Autodesk Inventor part; units mm, degrees
ref_plane "YZ Plane" through (0, 0, 0) normal (1, 0, 0) x (0, 1, 0)
ref_plane "XZ Plane" through (0, 0, 0) normal (0, 1, 0) x (-1, 0, 0)
ref_plane "XY Plane" through (0, 0, 0) normal (0, 0, 1) x (1, 0, 0)
sketch "Esquisse1" plane through (0, 0, 0) normal (0, 1, 0) x (-1, 0, 0)
  line L0 (21, 10.5) -> (-21, 10.5)
  line L1 (-21, 10.5) -> (-21, -10.5)
  line L2 (-21, -10.5) -> (21, -10.5)
  line L3 (21, -10.5) -> (21, 10.5)
  line L4 (29, 12.5) -> (-29, 12.5)
  line L5 (-29, 12.5) -> (-29, -12.5)
  line L6 (-29, -12.5) -> (29, -12.5)
  line L7 (29, -12.5) -> (29, 12.5)
  point P0 (0, 0)
  dimension "d0" = 21
  dimension "d1" = 10.5
  dimension "d2" = 42
  dimension "d3" = 21
  dimension "d4" = 2
  dimension "d5" = 2
  dimension "d6" = 8
  dimension "d7" = 8
extrude "Extrusion1" add sketch "Esquisse1" along normal blind 28
sketch "Esquisse2" plane through (0, 28, 0) normal (0, 1, 0) x (1, 0, 0)
  line L0 (-29, -12.5) -> (29, -12.5)
  line L1 (29, -12.5) -> (29, 12.5)
  line L2 (29, 12.5) -> (-29, 12.5)
  line L3 (-29, 12.5) -> (-29, -12.5)
  point P0 (0, 0)
extrude "Extrusion2" add sketch "Esquisse2" along normal blind 5
sketch "Esquisse3" plane through (0, 0, 0) normal (0, -1, 0) x (1, 0, 0)
  line L0 (-28, 10.5) -> (-21, 0) construction
  line L1 (-21, 0) -> (-28, -10.5) construction
  line L2 (-21, -10.5) -> (-28, 0) construction
  line L3 (-28, 0) -> (-21, 10.5) construction
  line L4 (21, 10.5) -> (28, 0) construction
  line L5 (21, -10.5) -> (28, 0) construction
  line L6 (28, -10.5) -> (21, 0) construction
  line L7 (21, 0) -> (28, 10.5) construction
  circle A0 centre (24.5, 5.25) radius 2
  circle A1 centre (24.5, -5.25) radius 2
  circle A2 centre (-24.5, 5.25) radius 2
  circle A3 centre (-24.5, -5.25) radius 2
  line L8 (-21, 10.5) -> (-28, 10.5)
  line L9 (-28, 10.5) -> (-28, -10.5)
  line L10 (-28, -10.5) -> (-21, -10.5)
  line L11 (-21, -10.5) -> (-21, 10.5)
  line L12 (28, 10.5) -> (21, 10.5)
  line L13 (21, 10.5) -> (21, -10.5)
  line L14 (21, -10.5) -> (28, -10.5)
  line L15 (28, -10.5) -> (28, 10.5)
  line L16 (21, 10.5) -> (21, -10.5)
  line L17 (21, -10.5) -> (-21, -10.5)
  line L18 (-21, 10.5) -> (21, 10.5)
  line L19 (-21, -10.5) -> (-21, 10.5)
  point P0 (0, 0)
  dimension "d12" = 4
  dimension "d13" = 4
  dimension "d14" = 4
  dimension "d15" = 4
  dimension "d25" = 7
  dimension "d26" = 7
extrude "Extrusion3" cut sketch "Esquisse3" against normal through all contours A0 | A1 | A2 | A3
sketch "Esquisse4" plane through (0, 28, 0) normal (0, -1, 0) x (1, 0, 0)
  line L0 (-21, 10.5) -> (10, 10.5)
  line L1 (10, 10.5) -> (10, -10.5)
  line L2 (10, -10.5) -> (-21, -10.5)
  line L3 (-21, -10.5) -> (-21, 10.5)
  line L4 (21, -10.5) -> (-21, -10.5)
  circle A0 centre (10, 0) radius 3.5
  line L5 (21, 10.5) -> (21, -10.5)
  point P0 (0, 0)
  dimension "d19" = 7
  dimension "d50" = 11
extrude "Extrusion4" cut sketch "Esquisse4" against normal through all contours A0 L1 | L1 A0
chamfer "Chanfrein1" distance 3 angle 45 1 edges at (6.5, 28, 0)
sketch "Esquisse5" plane through (-29, 0, 12.5) normal (0, 0, 1) x (1, 0, 0)
  line L0 (0, 0) -> (25, 0)
  line L1 (25, 0) -> (25, 19)
  line L2 (25, 19) -> (0, 19)
  line L3 (0, 19) -> (0, 0)
  line L4 (25, 0) -> (58, 0)
  line L5 (58, 0) -> (58, 6)
  line L6 (58, 6) -> (25, 6)
  line L7 (25, 6) -> (25, 0)
  line L8 (25, 19) -> (38, 6)
  point P0 (29, 0)
  dimension "d27" = 19
  dimension "d29" = 6
  dimension "d30" = 45
  dimension "d33" = 20
extrude "Extrusion5" cut sketch "Esquisse5" against normal through all
sketch "Esquisse6" plane through (0, 33, 0) normal (0, 1, 0) x (1, 0, 0)
  circle A0 centre (-24.5, -5.25) radius 4
  circle A1 centre (-24.5, 5.25) radius 4
  circle A2 centre (24.5, -5.25) radius 4
  circle A3 centre (24.5, 5.25) radius 4
  circle A4 centre (24.5, 5.25) radius 2
  circle A5 centre (24.5, -5.25) radius 2
  circle A6 centre (-24.5, -5.25) radius 2
  circle A7 centre (-24.5, 5.25) radius 2
  point P0 (0, 0)
  dimension "d34" = 8
  dimension "d35" = 8
  dimension "d36" = 8
  dimension "d37" = 8
extrude "Extrusion6" cut sketch "Esquisse6" against normal blind 13
sketch "Esquisse7" plane through (29, 33, 12.5) normal (1, 0, 0) x (0, 0, -1)
  line L0 (7.5, -27) -> (17.5, -27)
  line L1 (17.5, -27) -> (17.5, -5)
  line L2 (17.5, -5) -> (7.5, -5)
  line L3 (7.5, -5) -> (7.5, -27)
  line L4 (0, -27) -> (25, -27)
  line L5 (15.8135, -5) -> (9.1865, -5)
  line L6 (17.5, -27) -> (15.5, -27)
  line L7 (15.5, -27) -> (15.5, -17)
  line L8 (15.5, -17) -> (17.5, -17)
  line L9 (17.5, -17) -> (17.5, -27)
  line L10 (7.5, -27) -> (9.5, -27)
  line L11 (9.5, -27) -> (9.5, -17)
  line L12 (9.5, -17) -> (7.5, -17)
  line L13 (7.5, -17) -> (7.5, -27)
  point P0 (12.5, -33)
  dimension "d40" = 10
  dimension "d41" = 5
  dimension "d44" = 6
  dimension "d45" = 3
  dimension "d46" = 10
extrude "Extrusion7" cut sketch "Esquisse7" against normal up to next contours L11 L12 L3 L2 L1 L8 L7 L0
chamfer "Chanfrein2" distance 2 angle 45 2 edges at (25, 16, 3) (25, 16, -3)
sketch "Esquisse8" plane through (0, 28, 0) normal (0, -1, 0) x (1, 0, 0)
  line L0 (-16, -5.5) -> (-1.5, -5.5)
  line L1 (-1.5, -5.5) -> (-1.5, 5.5)
  line L2 (-1.5, 5.5) -> (-16, 5.5)
  line L3 (-16, 5.5) -> (-16, -5.5)
  line L4 (-21, 3.3135) -> (-21, -3.3135)
  line L5 (-4, 10.5) -> (-21, 10.5)
  line L6 (-21, -10.5) -> (-4, -10.5)
  circle A0 centre (10, 0) radius 6.5
  point P0 (0, 0)
  dimension "d51" = 5
  dimension "d52" = 5
  dimension "d53" = 5
  dimension "d54" = 5
extrude "Extrusion8" cut sketch "Esquisse8" against normal through all contours L3 L2 L1 L0
chamfer "Chanfrein3" distance 3 angle 45 4 edges at (-8.75, 33, 5.5) (-1.5, 33, 0) (-8.75, 33, -5.5) (-16, 33, 0)
equation "\"d13\" = d12"
equation "\"d14\" = d12"
equation "\"d15\" = d12"
equation "\"d35\" = d34"
equation "\"d36\" = d34"
equation "\"d37\" = d34"
properties part number "forearm_anti_axe"
Geometry: final body of the model. Coordinates: model frame, mm. A direction names the side the tool comes from. Round coordinates to 2 decimals unless told otherwise and drop trailing zeros. Order: outer loops, then holes, each group sorted by start corner. A loop starts at its lowest first (then second) coordinate and runs counter-clockwise, first axis right, second up.
Q1. Material intervals for probe 1 along Z at (x, y) = (-24.5, 19.65); probe 2 along X at (y, z) = (30, 5.25); probe 3 along X at (y, z) = (27.5, 5.25), sorted ascending.
Result sheet:
probe 1: z = -12.5 to -7.25, -3.25 to 3.25, 7.25 to 12.5
probe 2: x = -29 to -28.5, -20.5 to -16, -1.5 to 20.5, 28.5 to 29
probe 3: x = -29 to -28.5, 28.5 to 29
Q2. Section C-C, the plane y = 18. Output: boundary loops of the cut face in (x, z).
Result sheet:
outline: (-3, -12.5) - (29, -12.5) - (29, -5) - (26.48, -5) arc R2 cw (long way) to (22.52, -5) - (21, -5) - (21, -10.5) - (-3, -10.5) - close; (-3, 10.5) - (21, 10.5) - (21, 5) - (22.52, 5) arc R2 cw (long way) to (26.48, 5) - (29, 5) - (29, 12.5) - (-3, 12.5) - close
Q3. Pin query (flat end, axial travel): pin 1 (8 mm diameter, centred on y = 9.5, z = 7.5, fed in from -X); pin 2 (6.5 mm diameter, centred on x = -6.5, y = 15, fed in from -Z); pin 3 (12.5 mm diameter, centred on x = -18.5, z = 6, fed in from -Y); pin 4 (4 mm diameter, centred on x = -24, z = -4.5, fed in from +Y). Return the tip coordinate at first contact, or that it passes through.
Result sheet:
pin 1: stops at x = 2.85
pin 2: passes through
pin 3: stops at y = 19
pin 4: stops at y = 20
Q4. Section D-D, the plane z = 0. Output: boundary loops of the cut face in (x, y), and give its area (4 significant figures).
Result sheet:
outline: (-29, 19) - (-21, 19) - (-21, 28) - (-16, 28) - (-16, 30) - (-19, 33) - (-29, 33) - close; (-1.5, 28) - (3.5, 28) - (6.5, 31) - (6.5, 33) - (1.5, 33) - (-1.5, 30) - close; (13.5, 31) - (16.5, 28) - (29, 28) - (29, 33) - (13.5, 33) - close
area: 236.5 mm2
Q5. Section A-A, the plane y = 12.75. Output: boundary loops of the cut face in (x, z).
Result sheet:
outline: (2.25, -12.5) - (29, -12.5) - (29, -3) - (21, -3) - (21, -10.5) - (2.25, -10.5) - close; (2.25, 10.5) - (21, 10.5) - (21, 3) - (29, 3) - (29, 12.5) - (2.25, 12.5) - close; hole circle Ø4 at (24.5, -5.25); hole circle Ø4 at (24.5, 5.25)
Q6. Section B-B, the plane x = -24.5. Output: boundary loops of the cut face in (y, z).
Result sheet:
outline: (19, -12.5) - (33, -12.5) - (33, -9.25) - (20, -9.25) - (20, -7.25) - (19, -7.25) - close; (19, -3.25) - (20, -3.25) - (20, -1.25) - (33, -1.25) - (33, 1.25) - (20, 1.25) - (20, 3.25) - (19, 3.25) - close; (19, 7.25) - (20, 7.25) - (20, 9.25) - (33, 9.25) - (33, 12.5) - (19, 12.5) - close
Q7. Access query for faces 1 (the face through (25.9, 14.5, 3.5)), 2 (the face through (4, 19, 10.5)), 3 (the face through (25, 20, -8)), 4 (the face through (-1.5, 29, 0)), 5 (the face through (-22, 19, 0)). Directions: +Z, -Z, +X, -X, +Y, -Y. A direction counts if a zero-diameter tool reaches every point of the face in a straight line with its end or side. Return the directions, or none.
Result sheet:
face 1: +X, -X
face 2: -Y
face 3: +Y
face 4: +Y, -Y
face 5: +Z, -Z, -X, -Y
Q8. Mould query, pull axis Z, two halves, no side actions, for faces 6 (the face through (22, 18, 5)), 7 (the face through (21.4, 6, -8.7)). Classes: released by +Z, released by -Z, zero draft, split by the parting line, or undercut.
Result sheet:
face 6: undercut
face 7: zero draft
